from build123d import *

# Parameters (mm, degrees)
SKETCH3_R          = 1
CUT_EXTRUDE1_DEPTH = 4
SKETCH4_R          = 1
CUT_EXTRUDE2_DEPTH = 3


with BuildPart() as part:
    # Sketch2 → Revolve2 (revolve)
    with BuildSketch(Plane.XY):
        Polygon((1, 23.8), (0, 23.8), (0, 0), (1, 0), (1, 1.8), (9.5, 1.8), (11.5, 3.8), (11.5, 4.8), (11, 4.8), (11, 5.3), (11.5, 5.3), (11.5, 6.3), (9.5, 6.3), (9.5, 6.6), (11.5, 6.6), (11.5, 16.3), (7.5, 20.3), (1, 20.3), align=None)
    revolve(axis=Axis((0, 23.8, 0), (0, -1, 0)))

    # Sketch3 → Cut-Extrude1 (cut)
    with BuildSketch(Plane(origin=(0, 20.3, 0), x_dir=(1, 0, 0), z_dir=(0, 1, 0))):
        with Locations((0, 4.5)):
            Circle(SKETCH3_R)
        with Locations((0, -4.5)):
            Circle(SKETCH3_R)
        with Locations((4.5, 0)):
            Circle(SKETCH3_R)
        with Locations((-4.5, 0)):
            Circle(SKETCH3_R)
        with BuildLine():
            Line((-3, 9), (-3, 17.274276686))
            Line((-3, 17.274276686), (3, 17.274276686))
            Line((3, 17.274276686), (3, 9))
            ThreePointArc((3, 9), (0, 6), (-3, 9))
        make_face()
        with BuildLine():
            Line((13.459962442, 11.235214554), (16.459962442, 6.039062131))
            Line((16.459962442, 6.039062131), (9.294228634, 1.901923789))
            ThreePointArc((9.294228634, 1.901923789), (5.196152423, 3), (6.294228634, 7.098076211))
            Line((6.294228634, 7.098076211), (13.459962442, 11.235214554))
        make_face()
        with BuildLine():
            Line((16.459962442, -6.039062131), (13.459962442, -11.235214554))
            Line((13.459962442, -11.235214554), (6.294228634, -7.098076211))
            ThreePointArc((6.294228634, -7.098076211), (5.196152423, -3), (9.294228634, -1.901923789))
            Line((9.294228634, -1.901923789), (16.459962442, -6.039062131))
        make_face()
        with BuildLine():
            Line((3, -17.274276686), (-3, -17.274276686))
            Line((-3, -17.274276686), (-3, -9))
            ThreePointArc((-3, -9), (0, -6), (3, -9))
            Line((3, -9), (3, -17.274276686))
        make_face()
        with BuildLine():
            Line((-13.459962442, -11.235214554), (-16.459962442, -6.039062131))
            Line((-16.459962442, -6.039062131), (-9.294228634, -1.901923789))
            ThreePointArc((-9.294228634, -1.901923789), (-5.196152423, -3), (-6.294228634, -7.098076211))
            Line((-6.294228634, -7.098076211), (-13.459962442, -11.235214554))
        make_face()
        with BuildLine():
            Line((-16.459962442, 6.039062131), (-13.459962442, 11.235214554))
            Line((-13.459962442, 11.235214554), (-6.294228634, 7.098076211))
            ThreePointArc((-6.294228634, 7.098076211), (-5.196152423, 3), (-9.294228634, 1.901923789))
            Line((-9.294228634, 1.901923789), (-16.459962442, 6.039062131))
        make_face()
    extrude(amount=-CUT_EXTRUDE1_DEPTH, mode=Mode.SUBTRACT)

    # Sketch4 → Cut-Extrude2 (cut)
    with BuildSketch(Plane.XZ.offset(-1.8)):
        with Locations((0, 6)):
            Circle(SKETCH4_R)
        with Locations((8, 0)):
            Circle(SKETCH4_R)
        with Locations((0, -6)):
            Circle(SKETCH4_R)
        with Locations((-8, 0)):
            Circle(SKETCH4_R)
    extrude(amount=-CUT_EXTRUDE2_DEPTH, mode=Mode.SUBTRACT)


solid = part.part
Model file for the job. Use its own axes, mm. A direction names the side the tool comes from. Give positions to 0.01 mm unless a question says otherwise; leave off trailing zeros. Write each loop counter-clockwise with the first axis right and the second up, starting at its lowest first coordinate (ties: lowest second). Pieces come first, ordered by that corner, then holes. Notation, with made-up numbers: M 54.25,64.5 L 83.25,64.5 A28 cw 83.25,82.5 Z; hole C 9,-25.5 d6. An arc over 180 degrees is marked long. One line per item, written item: value. Start each with the question number.
Q1. 3-axis set-ups, long thin cutter, end or side, ignore diameter. For faces 4 (the cylindrical face through (4.38, 6.45, -8.43)), 5 (the cylindrical face through (0, 3, 7)), 6 (the cylindrical face through (-5.3, 18.3, 0.6)), 7 (the flat face through (-6.813, 16.873, -7.397)): which of +Z, -Z, +X, -X, +Y, -Y reach the whole face in a straight line?
Q2. Probe probe 1 along Z at (x, y) = (0, 18.55); probe 2 along Z at (x, y) = (0, 2.6); probe 3 along X at (y, z) = (18.85, 0). List the from-to ranges inside material, lowest first. Write a range as [from, to].
Q3. Saw through at C-C, the plane y = 19.75. Write the cut outline in (x, z), plus the area to 3 significant figures.
Q4. Saw through at B-B, the plane y = 8.5. Write the cut outline in (x, z).
Q5. Drop flat-ended pins along their axis: pin 1 Ø1.6 at (x, z) = (0, 4.5) entering from +Y; pin 2 Ø2.5 at (x, z) = (0, 6) entering from +Y; pin 3 Ø2 at (y, z) = (17.5, -10) entering from +X. Give the stop position or say it passes through.
Q6. Two-plate mould, pull along Z, no slides. Class faces 1 (the cylindrical face through (3.5, 18.3, 0)), 2 (the cylindrical face through (0, 22, -1)), 3 (the flat face through (2, 20.3, 0)): +Z half, -Z half, draft (parallel to the pull), parting line (faces both ways), or undercut.
Q7. Saw through at A-A, the plane y = 17.25. Write the cut outline in (x, z).
Output values:
1. face 4: none
1. face 5: -Y
1. face 6: +Y
1. face 7: -X, +Y
2. probe 1: z = [-6, -5.5], [-3.5, 3.5], [5.5, 6]
2. probe 2: z = [-10.3, -7], [-5, 5], [7, 10.3]
2. probe 3: x = [-8.95, -5.5], [-3.5, 3.5], [5.5, 8.95]
3. outline: M -7.91,-1.5 A3 cw -5.26,-6.1 A8.05 ccw -2.65,-7.6 A3 cw 2.65,-7.6 A8.05 ccw 5.26,-6.1 A3 cw 7.91,-1.5 A8.05 ccw 7.91,1.5 A3 cw 5.26,6.1 A8.05 ccw 2.65,7.6 A3 cw -2.65,7.6 A8.05 ccw -5.26,6.1 A3 cw -7.91,1.5 A8.05 ccw Z; hole C -4.5,0 d2; hole C 0,-4.5 d2; hole C 0,4.5 d2; hole C 4.5,0 d2
3. area: 145 mm²
4. outline: C 0,0 d23
5. pin 1: stops at y = 16.3
5. pin 2: stops at y = 20.3
5. pin 3: stops at x = 5.91
6. face 1: undercut
6. face 2: parting line
6. face 3: draft
7. outline: M -10.26,-2.46 L -9.29,-1.9 A3 cw -6.29,-7.1 L -7.26,-7.66 A10.55 ccw -3,-10.11 L -3,-9 A3 cw 3,-9 L 3,-10.11 A10.55 ccw 7.26,-7.66 L 6.29,-7.1 A3 cw 9.29,-1.9 L 10.26,-2.46 A10.55 ccw 10.26,2.46 L 9.29,1.9 A3 cw 6.29,7.1 L 7.26,7.66 A10.55 ccw 3,10.11 L 3,9 A3 cw -3,9 L -3,10.11 A10.55 ccw -7.26,7.66 L -6.29,7.1 A3 cw -9.29,1.9 L -10.26,2.46 A10.55 ccw Z; hole C -4.5,0 d2; hole C 0,-4.5 d2; hole C 0,4.5 d2; hole C 4.5,0 d2
